Work out the finished part from the listing and answer in its coordinate system (mm). Give positions to 0.01 mm unless a question says otherwise; leave off trailing zeros. Loops run counter-clockwise (first coordinate to the right, second up) from the corner with the lowest first, then second, coordinate; pieces in that order, holes last. Notation, with made-up numbers: (9, 85) - (68, 85) arc R23 cw to (68, 111) - close; hole circle Ø5 at (46.5, 36.25). An arc over 180 degrees is marked (long way). Use CSV: the item, a comma, the result in double quotes.
from build123d import *


with BuildPart() as f1:
    # F0 (on Right) → F1 (revolve)
    with BuildSketch(Plane.YZ):
        Polygon((-12, 0), (-6.4, 0), (-6.4, 2), (-6.4, 2.2704), (-12, 2.2704), align=None)
        with BuildLine():
            Line((-6.4, 2), (-6.4, 0))
            Line((-6.4, 0), (-5.975, 0.425))
            Line((-5.975, 0.425), (-5.975, 1.575))
            ThreePointArc((-5.975, 1.575), (-6.09948, 1.87552), (-6.4, 2))
        make_face()
    revolve(axis=Axis((0, 0, 18.057704), (0, 0, 1)))


solid = f1.part
Item 1: The mould has two halves that part along X. Classify faces 1 (the cylindrical face through (5.04, -3.21, 1.01)), 2 (the cylindrical face through (0.53, 11.99, 1.12)), 3 (the flat face through (-5, 5, 2.27)): pulls with the +X half, pulls with the -X half, needs draft (parallel to the pull), parting line crosses it, or undercut.
Determined:
face 1,"undercut"
face 2,"parting line crosses it"
face 3,"needs draft"
Item 2: Given P1, Ø9.5, axis at x = 0, y = 0, coming from the -Z side, flat-ended and moving along its own axis, determine where the tip first touches the part or whether it passes through.
Determined:
P1,"passes through"
Item 3: A cutting plane is placed at C-C on z = 1.15. Determine the outline of the cut face in (x, y) (3 decimals), and give its area (3 significant figures).
Determined:
outline,"circle Ø24 at (0, 0); hole circle Ø11.95 at (0, 0)"
area,"340 mm²"
Item 4: A cutting plane is placed at A-A on x = 0. Determine the outline of the cut face in (y, z) (3 decimals), and give its area (3 significant figures).
Determined:
outline,"(-12, 0) - (-6.4, 0) - (-5.975, 0.425) - (-5.975, 1.575) arc R0.425 ccw to (-6.4, 2) - (-6.4, 2.27) - (-12, 2.27) - close; (5.975, 0.425) - (6.4, 0) - (12, 0) - (12, 2.27) - (6.4, 2.27) - (6.4, 2) arc R0.425 ccw to (5.975, 1.575) - close"
area,"26.9 mm²"
Item 5: Find the intervals of material crossed by line 1 (X direction, y = 0, z = 2.15); line 2 (X direction, y = 0, z = 1.3) (3 decimals); line 3 (Y direction, x = -3, z = 1.05), in increasing order.
Determined:
line 1,"x = -12 to -6.4, 6.4 to 12"
line 2,"x = -12 to -5.975, 5.975 to 12"
line 3,"y = -11.62 to -5.17, 5.17 to 11.62"
Item 6: A cutting plane is placed at D-D on y = -8.75. Determine the outline of the cut face in (x, z), and give its area (3 significant figures).
Determined:
outline,"(-8.21, 0) - (8.21, 0) - (8.21, 2.27) - (-8.21, 2.27) - close"
area,"37.3 mm²"
